```python
from build123d import *

# Parameters (mm, degrees)
F0_R     = 11
F1_DEPTH = 3.5


with BuildPart() as f1:
    # F0 (on Top) → F1 (new body, symmetric)
    with BuildSketch(Plane.XY):
        with BuildLine():
            Line((-2.5, 13.774977314), (-2.5, 16.225022686))
            ThreePointArc((-2.5, 16.225022686), (0, 16), (2.5, 16.225022686))
            Line((2.5, 16.225022686), (2.5, 13.774977314))
            ThreePointArc((2.5, 13.774977314), (3.7662181175, 13.483901553), (5, 13.0766968306))
            Line((5, 13.0766968306), (5, 16.9233031694))
            ThreePointArc((5, 16.9233031694), (0, 44), (-5, 16.9233031694))
            Line((-5, 16.9233031694), (-5, 13.0766968306))
            ThreePointArc((-5, 13.0766968306), (-3.7662181175, 13.483901553), (-2.5, 13.774977314))
        make_face()
        with Locations((0, 30)):
            Circle(F0_R, mode=Mode.SUBTRACT)
        with BuildLine():
            ThreePointArc((2.5, 13.774977314), (0, 14), (-2.5, 13.774977314))
            ThreePointArc((-2.5, 13.774977314), (-3.7662181175, 13.483901553), (-5, 13.0766968306))
            ThreePointArc((-5, 13.0766968306), (-9.3853246706, 10.3882472452), (-12.503686361, 6.2974461002))
            ThreePointArc((-12.503686361, 6.2974461002), (-11.3865869691, 3.2363861749), (-11.007372722, 0))
            ThreePointArc((-11.007372722, 0), (-11.3865869691, -3.2363861749), (-12.503686361, -6.2974461002))
            ThreePointArc((-12.503686361, -6.2974461002), (-9.3853246706, -10.3882472452), (-5, -13.0766968306))
            ThreePointArc((-5, -13.0766968306), (-3.7662181175, -13.483901553), (-2.5, -13.774977314))
            ThreePointArc((-2.5, -13.774977314), (0, -14), (2.5, -13.774977314))
            ThreePointArc((2.5, -13.774977314), (3.7662181175, -13.483901553), (5, -13.0766968306))
            ThreePointArc((5, -13.0766968306), (9.3853246706, -10.3882472452), (12.503686361, -6.2974461002))
            ThreePointArc((12.503686361, -6.2974461002), (11.007372722, 0), (12.503686361, 6.2974461002))
            ThreePointArc((12.503686361, 6.2974461002), (9.3853246706, 10.3882472452), (5, 13.0766968306))
            ThreePointArc((5, 13.0766968306), (3.7662181175, 13.483901553), (2.5, 13.774977314))
        make_face()
        Circle(F0_R, mode=Mode.SUBTRACT)
        with BuildLine():
            ThreePointArc((-12.503686361, -6.2974461002), (-14, 0), (-12.503686361, 6.2974461002))
            ThreePointArc((-12.503686361, 6.2974461002), (-39.007372722, 0), (-12.503686361, -6.2974461002))
        make_face()
        with Locations((-25.007372722, 0)):
            Circle(F0_R, mode=Mode.SUBTRACT)
        with BuildLine():
            ThreePointArc((-11.007372722, 0), (-11.3865869691, 3.2363861749), (-12.503686361, 6.2974461002))
            ThreePointArc((-12.503686361, 6.2974461002), (-14, 0), (-12.503686361, -6.2974461002))
            ThreePointArc((-12.503686361, -6.2974461002), (-11.3865869691, -3.2363861749), (-11.007372722, 0))
        make_face()
        with BuildLine():
            ThreePointArc((12.503686361, -6.2974461002), (14, 0), (12.503686361, 6.2974461002))
            ThreePointArc((12.503686361, 6.2974461002), (11.007372722, 0), (12.503686361, -6.2974461002))
        make_face()
        with BuildLine():
            ThreePointArc((39.007372722, 0), (28.2437588969, 13.6207857529), (12.503686361, 6.2974461002))
            ThreePointArc((12.503686361, 6.2974461002), (14, 0), (12.503686361, -6.2974461002))
            ThreePointArc((12.503686361, -6.2974461002), (28.2437588969, -13.6207857529), (39.007372722, 0))
        make_face()
        with Locations((25.007372722, 0)):
            Circle(F0_R, mode=Mode.SUBTRACT)
        with BuildLine():
            ThreePointArc((-2.5, -13.774977314), (-3.7662181175, -13.483901553), (-5, -13.0766968306))
            Line((-5, -13.0766968306), (-5, -16.9233031694))
            ThreePointArc((-5, -16.9233031694), (0, -44), (5, -16.9233031694))
            Line((5, -16.9233031694), (5, -13.0766968306))
            ThreePointArc((5, -13.0766968306), (3.7662181175, -13.483901553), (2.5, -13.774977314))
            Line((2.5, -13.774977314), (2.5, -16.225022686))
            ThreePointArc((2.5, -16.225022686), (0, -16), (-2.5, -16.225022686))
            Line((-2.5, -16.225022686), (-2.5, -13.774977314))
        make_face()
        with Locations((0, -30)):
            Circle(F0_R, mode=Mode.SUBTRACT)
    extrude(amount=F1_DEPTH, both=True)


solid = f1.part
```
Geometry check sheet. Reference: the model listing, model coordinates, mm. A direction names the side the tool comes from. Give positions to 0.01 mm unless a question says otherwise; leave off trailing zeros. Order: outer loops, then holes, each group sorted by start corner. A loop starts at its lowest first (then second) coordinate and runs counter-clockwise, first axis right, second up.
1. Thickness scan on L1, parallel to X at y = 1, z = 2.5; L2, parallel to X at y = 7, z = -1.5; L3, parallel to X at y = -5.5, z = -1. Record the ranges inside material, lowest first.
2. Release check for a two-part mould opening along Y. For faces 1 (the face through (9.44, 10.34, 0.05)), 2 (the face through (6, -10, 3.5)), 3 (the face through (-9.33, 10.44, 0.05)) record: pulls with the +Y half, pulls with the -Y half, needs draft (parallel to the pull), parting line crosses it, or undercut.
3. Section check C-C, the plane y = 21. Enter the section's corners in (x, z), and give its area (3 significant figures).
4. Section check A-A, the plane x = 0. Enter the section's corners in (y, z).
5. Section check D-D, the plane y = -10. Enter the section's corners in (x, z), and give its area (3 significant figures).
6. Gauge pin test, flat ends, axial feed: pin 1 Ø17.5 at (x, y) = (25.01, 0) entering from -Z; pin 2 Ø1.2 at (y, z) = (15, 1) entering from -X; pin 3 Ø3 at (x, z) = (-27.5, -0.5) entering from -Y; pin 4 Ø0.7 at (y, z) = (15, -1.5) entering from +X. Record the tip position at first contact, or that the pin passes through.
7. Access from +Z, -Z, +X, -X, +Y, -Y to the whole of each face (thin tool, end or side, straight path). Record for faces 4 (the face through (6, -10, -3.5)), 5 (the face through (-5, 15, 0)).
8. Section check B-B, the plane z = 1. Enter the section's corners in (x, y).
Values follow:
1. L1: x = -38.97 to -35.96, -14.05 to -10.95, 10.95 to 14.05, 35.96 to 38.97
1. L2: x = -37.13 to -33.49, -16.52 to -12.88, -12.12 to -8.49, 8.49 to 12.12, 12.88 to 16.52, 33.49 to 37.13
1. L3: x = -37.88 to -34.53, -15.48 to -9.53, 9.53 to 15.48, 34.53 to 37.88
2. face 1: undercut
2. face 2: needs draft
2. face 3: undercut
3. outline: (-10.72, -3.5) - (-6.32, -3.5) - (-6.32, 3.5) - (-10.72, 3.5) - close; (6.32, -3.5) - (10.72, -3.5) - (10.72, 3.5) - (6.32, 3.5) - close
3. area: 61.6 mm2
4. outline: (-44, -3.5) - (-41, -3.5) - (-41, 3.5) - (-44, 3.5) - close; (-19, -3.5) - (-16, -3.5) - (-16, 3.5) - (-19, 3.5) - close; (-14, -3.5) - (-11, -3.5) - (-11, 3.5) - (-14, 3.5) - close; (11, -3.5) - (14, -3.5) - (14, 3.5) - (11, 3.5) - close; (16, -3.5) - (19, -3.5) - (19, 3.5) - (16, 3.5) - close; (41, -3.5) - (44, -3.5) - (44, 3.5) - (41, 3.5) - close
5. outline: (-34.81, -3.5) - (-29.59, -3.5) - (-29.59, 3.5) - (-34.81, 3.5) - close; (-20.42, -3.5) - (-15.21, -3.5) - (-15.21, 3.5) - (-20.42, 3.5) - close; (-9.8, -3.5) - (-4.58, -3.5) - (-4.58, 3.5) - (-9.8, 3.5) - close; (4.58, -3.5) - (9.8, -3.5) - (9.8, 3.5) - (4.58, 3.5) - close; (15.21, -3.5) - (20.42, -3.5) - (20.42, 3.5) - (15.21, 3.5) - close; (29.59, -3.5) - (34.81, -3.5) - (34.81, 3.5) - (29.59, 3.5) - close
5. area: 219 mm2
6. pin 1: passes through
6. pin 2: stops at x = -5
6. pin 3: stops at y = -13.96
6. pin 4: stops at x = 5
7. face 4: -Z, +X, -X, +Y, -Y
7. face 5: +Z, -Z
8. outline: (-12.5, -6.3) arc R14 ccw to (-5, -13.08) - (-5, -16.92) arc R14 ccw (long way) to (5, -16.92) - (5, -13.08) arc R14 ccw to (12.5, -6.3) arc R14 ccw (long way) to (12.5, 6.3) arc R14 ccw to (5, 13.08) - (5, 16.92) arc R14 ccw (long way) to (-5, 16.92) - (-5, 13.08) arc R14 ccw to (-12.5, 6.3) arc R14 ccw (long way) to start; hole circle Ø22 at (-25.01, 0); hole circle Ø22 at (0, -30); hole circle Ø22 at (0, 0); hole circle Ø22 at (0, 30); hole (-2.5, -16.23) arc R14 cw to (2.5, -16.23) - (2.5, -13.77) arc R14 cw to (-2.5, -13.77) - close; hole (-2.5, 13.77) arc R14 cw to (2.5, 13.77) - (2.5, 16.23) arc R14 cw to (-2.5, 16.23) - close; hole circle Ø22 at (25.01, 0)
